Build history of the part. All positions in model axes, mm. Give positions to 0.01 mm unless a question says otherwise; leave off trailing zeros. Write each loop counter-clockwise with the first axis right and the second up, starting at its lowest first coordinate (ties: lowest second). Pieces come first, ordered by that corner, then holes. Notation, with made-up numbers: (-19, 15) -> (-14, 15) arc R5 cw to (-14, 23) -> close; hole circle Ø9 at (24.25, -27.5). An arc over 180 degrees is marked (long way). Write item = value, one per line. Start each with the question number.
Q1. Wall check: line 1 (Y direction, x = 2, z = -38) (3 decimals); line 2 (Z direction, x = 22.5, y = 1641.5) (3 decimals); line 3 (Z direction, x = 1, y = 539). Give the ranges that are in metal, low to high.
Q2. Saw through at A-A, the plane y = 1464.5. List the corners of the cut face in (x, z) (3 decimals), then the cut area to 3 significant figures.
Q3. Drop flat-ended pins along their axis: P1, Ø7.5, axis at y = 730.25, z = -44.45, coming from the +X side (3 decimals); P2, Ø2, axis at x = 9, y = 368.5, coming from the -Z side (3 decimals). Give the stop position or say it passes through.
from build123d import *

# Parameters (mm, degrees)
BASE_FLANGE1_DEPTH = 2070.1
CUT_EXTRUDE1_DEPTH = 3.175
SKETCH3_R          = 3.429
SKETCH3_R_2        = 3.175
CUT_EXTRUDE2_DEPTH = 3.175
SKETCH4_R          = 3.429
SKETCH4_R_2        = 3.175
CUT_EXTRUDE3_DEPTH = 3.175
FILLET1_R          = 3.175


# Sheet-metal steps are written as plain solids
with BuildPart() as part:
    # Sketch1 → Base-Flange1 (new body)
    with BuildSketch(Plane(origin=(0, 0, 0), x_dir=(1, 0, 0), z_dir=(0, 1, 0))):
        with BuildLine():
            Line((50.8, 0), (6.35, 0))
            ThreePointArc((6.35, 0), (1.859871939, 1.859871939), (0, 6.35))
            Line((0, 6.35), (0, 50.8))
            Line((0, 50.8), (3.175, 50.8))
            Line((3.175, 50.8), (3.175, 6.35))
            ThreePointArc((3.175, 6.35), (4.10493597, 4.10493597), (6.35, 3.175))
            Line((6.35, 3.175), (50.8, 3.175))
            Line((50.8, 3.175), (50.8, 0))
        make_face()
    extrude(amount=BASE_FLANGE1_DEPTH)

    # Sketch2 → Cut-Extrude1 (cut)
    with BuildSketch(Plane(origin=(0, 2070.1, 0), x_dir=(1, 0, 0), z_dir=(0, 1, 0))):
        Polygon((6.35, 0), (0, 0), (0, 50.8), (6.35, 50.8), (6.35, 3.175), (50.8, 3.175), (50.8, 0), align=None)
    extrude(amount=-CUT_EXTRUDE1_DEPTH, mode=Mode.SUBTRACT)

    # Sketch3 → Cut-Extrude2 (cut)
    with BuildSketch(Plane.XY):
        with Locations((19.05, 2057.4)):
            Circle(SKETCH3_R)
        with Locations((19.05, 2038.35)):
            Circle(SKETCH3_R)
        with Locations((44.45, 1968.5)):
            Circle(SKETCH3_R_2)
        with Locations((44.45, 1949.45)):
            Circle(SKETCH3_R_2)
        with Locations((44.45, 1892.3)):
            Circle(SKETCH3_R_2)
        with Locations((44.45, 1873.25)):
            Circle(SKETCH3_R_2)
        with Locations((44.45, 1816.1)):
            Circle(SKETCH3_R_2)
        with Locations((44.45, 1797.05)):
            Circle(SKETCH3_R_2)
        with Locations((44.45, 1739.9)):
            Circle(SKETCH3_R_2)
        with Locations((44.45, 1720.85)):
            Circle(SKETCH3_R_2)
        with Locations((44.45, 1663.7)):
            Circle(SKETCH3_R_2)
        with Locations((44.45, 1644.65)):
            Circle(SKETCH3_R_2)
        with Locations((44.45, 1587.5)):
            Circle(SKETCH3_R_2)
        with Locations((44.45, 1568.45)):
            Circle(SKETCH3_R_2)
        with Locations((44.45, 1511.3)):
            Circle(SKETCH3_R_2)
        with Locations((44.45, 1492.25)):
            Circle(SKETCH3_R_2)
        with Locations((44.45, 1435.1)):
            Circle(SKETCH3_R_2)
        with Locations((44.45, 1416.05)):
            Circle(SKETCH3_R_2)
        with Locations((44.45, 1358.9)):
            Circle(SKETCH3_R_2)
        with Locations((44.45, 1339.85)):
            Circle(SKETCH3_R_2)
        with Locations((44.45, 1282.7)):
            Circle(SKETCH3_R_2)
        with Locations((44.45, 1263.65)):
            Circle(SKETCH3_R_2)
        with Locations((44.45, 1206.5)):
            Circle(SKETCH3_R_2)
        with Locations((44.45, 1187.45)):
            Circle(SKETCH3_R_2)
        with Locations((44.45, 1130.3)):
            Circle(SKETCH3_R_2)
        with Locations((44.45, 1111.25)):
            Circle(SKETCH3_R_2)
        with Locations((44.45, 1054.1)):
            Circle(SKETCH3_R_2)
        with Locations((44.45, 1035.05)):
            Circle(SKETCH3_R_2)
        with Locations((44.45, 977.9)):
            Circle(SKETCH3_R_2)
        with Locations((44.45, 958.85)):
            Circle(SKETCH3_R_2)
        with Locations((44.45, 901.7)):
            Circle(SKETCH3_R_2)
        with Locations((44.45, 882.65)):
            Circle(SKETCH3_R_2)
        with Locations((44.45, 825.5)):
            Circle(SKETCH3_R_2)
        with Locations((44.45, 806.45)):
            Circle(SKETCH3_R_2)
        with Locations((44.45, 749.3)):
            Circle(SKETCH3_R_2)
        with Locations((44.45, 730.25)):
            Circle(SKETCH3_R_2)
        with Locations((44.45, 596.9)):
            Circle(SKETCH3_R_2)
        with Locations((44.45, 577.85)):
            Circle(SKETCH3_R_2)
        with Locations((38.1, 546.1)):
            Circle(SKETCH3_R)
        with Locations((44.45, 673.1)):
            Circle(SKETCH3_R)
        with Locations((44.45, 654.05)):
            Circle(SKETCH3_R)
        with Locations((19.05, 539.75)):
            Circle(SKETCH3_R)
        with Locations((19.05, 520.7)):
            Circle(SKETCH3_R)
        with Locations((25.4, 15.875)):
            Circle(SKETCH3_R)
        with Locations((25.4, 34.925)):
            Circle(SKETCH3_R)
        with Locations((38.1, 527.05)):
            Circle(SKETCH3_R)
    extrude(amount=-CUT_EXTRUDE2_DEPTH, mode=Mode.SUBTRACT)

    # Sketch4 → Cut-Extrude3 (cut)
    with BuildSketch(Plane.ZY):
        with Locations((-19.05, 2057.4)):
            Circle(SKETCH4_R)
        with Locations((-19.05, 2038.35)):
            Circle(SKETCH4_R)
        with Locations((-44.45, 1968.5)):
            Circle(SKETCH4_R_2)
        with Locations((-44.45, 1949.45)):
            Circle(SKETCH4_R_2)
        with Locations((-44.45, 600.075)):
            Circle(SKETCH4_R_2)
        with Locations((-44.45, 581.025)):
            Circle(SKETCH4_R_2)
        with Locations((-38.1, 546.1)):
            Circle(SKETCH4_R)
        with Locations((-19.05, 539.75)):
            Circle(SKETCH4_R)
        with Locations((-44.45, 1873.25)):
            Circle(SKETCH4_R_2)
        with Locations((-44.45, 1892.3)):
            Circle(SKETCH4_R_2)
        with Locations((-44.45, 1797.05)):
            Circle(SKETCH4_R_2)
        with Locations((-44.45, 1816.1)):
            Circle(SKETCH4_R_2)
        with Locations((-44.45, 1720.85)):
            Circle(SKETCH4_R_2)
        with Locations((-44.45, 1739.9)):
            Circle(SKETCH4_R_2)
        with Locations((-44.45, 1644.65)):
            Circle(SKETCH4_R_2)
        with Locations((-44.45, 1663.7)):
            Circle(SKETCH4_R_2)
        with Locations((-44.45, 1568.45)):
            Circle(SKETCH4_R_2)
        with Locations((-44.45, 1587.5)):
            Circle(SKETCH4_R_2)
        with Locations((-44.45, 1492.25)):
            Circle(SKETCH4_R_2)
        with Locations((-44.45, 1511.3)):
            Circle(SKETCH4_R_2)
        with Locations((-44.45, 1416.05)):
            Circle(SKETCH4_R_2)
        with Locations((-44.45, 1435.1)):
            Circle(SKETCH4_R_2)
        with Locations((-44.45, 1339.85)):
            Circle(SKETCH4_R_2)
        with Locations((-44.45, 1358.9)):
            Circle(SKETCH4_R_2)
        with Locations((-44.45, 1263.65)):
            Circle(SKETCH4_R_2)
        with Locations((-44.45, 1282.7)):
            Circle(SKETCH4_R_2)
        with Locations((-44.45, 1187.45)):
            Circle(SKETCH4_R_2)
        with Locations((-44.45, 1206.5)):
            Circle(SKETCH4_R_2)
        with Locations((-44.45, 1111.25)):
            Circle(SKETCH4_R_2)
        with Locations((-44.45, 1130.3)):
            Circle(SKETCH4_R_2)
        with Locations((-44.45, 1035.05)):
            Circle(SKETCH4_R_2)
        with Locations((-44.45, 1054.1)):
            Circle(SKETCH4_R_2)
        with Locations((-44.45, 958.85)):
            Circle(SKETCH4_R_2)
        with Locations((-44.45, 977.9)):
            Circle(SKETCH4_R_2)
        with Locations((-44.45, 882.65)):
            Circle(SKETCH4_R_2)
        with Locations((-44.45, 901.7)):
            Circle(SKETCH4_R_2)
        with Locations((-44.45, 806.45)):
            Circle(SKETCH4_R_2)
        with Locations((-44.45, 825.5)):
            Circle(SKETCH4_R_2)
        with Locations((-44.45, 730.25)):
            Circle(SKETCH4_R_2)
        with Locations((-44.45, 749.3)):
            Circle(SKETCH4_R_2)
        with Locations((-44.45, 654.05)):
            Circle(SKETCH4_R_2)
        with Locations((-44.45, 673.1)):
            Circle(SKETCH4_R_2)
        with Locations((-19.05, 520.7)):
            Circle(SKETCH4_R)
        with Locations((-25.4, 34.925)):
            Circle(SKETCH4_R)
        with Locations((-25.4, 15.875)):
            Circle(SKETCH4_R)
        with Locations((-38.1, 527.05)):
            Circle(SKETCH4_R)
    extrude(amount=-CUT_EXTRUDE3_DEPTH, mode=Mode.SUBTRACT)

    # Fillet1
    fillet1_edges = [part.edges().sort_by_distance(p)[0] for p in [
        (1.5875, 2066.925, -50.8),
        (50.8, 2066.925, -1.5875),
        (1.5875, 0, -50.8),
        (50.8, 0, -1.5875),
    ]]
    fillet(fillet1_edges, radius=FILLET1_R)


solid = part.part
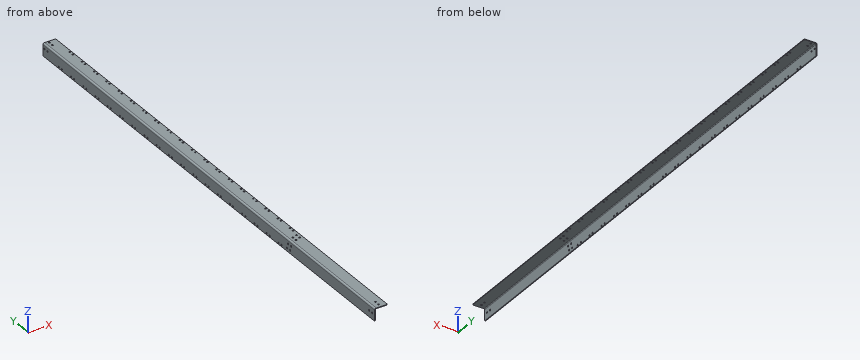
Report:
q1.line_1 = 0 to 523.622, 530.478 to 542.672, 549.528 to 2066.925
q1.line_2 = -3.175 to 0
q1.line_3 = -50.8 to -22.4, -15.7 to -2.93
q2.outline = (0, -50.8) -> (3.175, -50.8) -> (3.175, -6.35) arc R3.175 cw to (6.35, -3.175) -> (50.8, -3.175) -> (50.8, 0) -> (6.35, 0) arc R6.35 ccw to (0, -6.35) -> close
q2.area = 306 mm2
q3.P1 = 3.175
q3.P2 = -3.175
